Work out the finished part from the listing and answer in its coordinate system (mm). A direction names the side the tool comes from. Give positions to 0.01 mm unless a question says otherwise; leave off trailing zeros. Loops run counter-clockwise (first coordinate to the right, second up) from the corner with the lowest first, then second, coordinate; pieces in that order, holes last. Notation, with made-up numbers: (6, -0.75) -> (60, -0.75) arc R20 cw to (60, 23.25) -> close; hole circle Ø10 at (71.25, -9). An arc over 180 degrees is marked (long way). Answer as CSV lines item,"result". Start each with the question number.
1. Find section D-D, the plane x = 7.5. Give the vertices of the cut face in (y, z).
2. A tool of negligible diameter and unlimited length cuts with its end or side. For faces 5 (the face through (30.758, 2.465, -17.726)), 6 (the face through (2.74, 2.46, 33.43)), 7 (the face through (-27.522, 2.465, -19.077)), 8 (the face through (-30.282, 2.465, 14.296)), 9 (the face through (27.522, 2.465, 19.077)), from which of +Z, -Z, +X, -X, +Y, -Y can it reach the whole face along a straight path? Write none if from no direction.
3. Determine the mould class of faces 1 (the face through (15.59, 2.46, 27.37)), 2 (the face through (27.583, 2.465, -19.088)), 3 (the face through (30.32, 2.46, 14.34)), 4 (the face through (30.282, 2.465, -14.296)) for opening direction Z: +Z half, -Z half, draft (parallel to the pull), parting line (faces both ways), or undercut.
4. Find the intervals of material crossed by line 1 along X through (y, z) = (1.5, 20); line 2 along X through (y, z) = (3.45, -16); line 3 along Z through (x, y) = (-22, 0.25), in increasing order.
5. A flat-ended cylindrical pin translates along its axis: pin 1 Ø1.5 at (y, z) = (2, -2) entering from +X. Find the tip coordinate at first contact, or state that the pin passes through.
6. Find section C-C, the plane z = 4.5. Give the vertices of the cut face in (x, y), and give its area (3 significant figures).
7. Find section B-B, the plane x = 0. Give the vertices of the cut face in (y, z).
8. Find section A-A, the plane y = 3.7. Give the vertices of the cut face in (x, z), and give its area (3 significant figures).
from build123d import *

# Parameters (mm, degrees)
BOSS_EXTRUDE1_DEPTH = 5
SKETCH2_R           = 2.6
CUT_EXTRUDE1_DEPTH  = 5


with BuildPart() as part:
    # Sketch1 → Boss-Extrude1 (new body)
    with BuildSketch(Plane(origin=(0, 0, 0), x_dir=(1, 0, 0), z_dir=(0, 1, 0))):
        with BuildLine():
            Line((2, 35.5), (-2, 35.5))
            Line((-2, 35.5), (-3.5, 31.304951685))
            ThreePointArc((-3.5, 31.304951685), (-15.75, 27.279800219), (-25.360883423, 18.683564756))
            Line((-25.360883423, 18.683564756), (-29.743901834, 19.482050808))
            Line((-29.743901834, 19.482050808), (-31.743901834, 16.017949192))
            Line((-31.743901834, 16.017949192), (-28.860883423, 12.621386929))
            ThreePointArc((-28.860883423, 12.621386929), (-31.5, 0), (-28.860883423, -12.621386929))
            Line((-28.860883423, -12.621386929), (-31.743901834, -16.017949192))
            Line((-31.743901834, -16.017949192), (-29.743901834, -19.482050808))
            Line((-29.743901834, -19.482050808), (-25.360883423, -18.683564756))
            ThreePointArc((-25.360883423, -18.683564756), (-15.75, -27.279800219), (-3.5, -31.304951685))
            Line((-3.5, -31.304951685), (-2, -35.5))
            Line((-2, -35.5), (2, -35.5))
            Line((2, -35.5), (3.5, -31.304951685))
            ThreePointArc((3.5, -31.304951685), (15.75, -27.279800219), (25.360883423, -18.683564756))
            Line((25.360883423, -18.683564756), (29.743901834, -19.482050808))
            Line((29.743901834, -19.482050808), (31.743901834, -16.017949192))
            Line((31.743901834, -16.017949192), (28.860883423, -12.621386929))
            ThreePointArc((28.860883423, -12.621386929), (31.5, 0), (28.860883423, 12.621386929))
            Line((28.860883423, 12.621386929), (31.743901834, 16.017949192))
            Line((31.743901834, 16.017949192), (29.743901834, 19.482050808))
            Line((29.743901834, 19.482050808), (25.360883423, 18.683564756))
            ThreePointArc((25.360883423, 18.683564756), (15.75, 27.279800219), (3.5, 31.304951685))
            Line((3.5, 31.304951685), (2, 35.5))
        make_face()
    extrude(amount=BOSS_EXTRUDE1_DEPTH)

    # Sketch2 → Cut-Extrude1 (cut)
    with BuildSketch(Plane(origin=(0, 5, 0), x_dir=(1, 0, 0), z_dir=(0, 1, 0))):
        with Locations(Location((0, 20, 0), (0, 0, 270))):
            Circle(SKETCH2_R)
        with Locations(Location((0, -20, 0), (0, 0, 90))):
            Circle(SKETCH2_R)
    extrude(amount=-CUT_EXTRUDE1_DEPTH, mode=Mode.SUBTRACT)


solid = part.part
Resolved:
1,outline,"(0, -30.59) -> (5, -30.59) -> (5, 30.59) -> (0, 30.59) -> close"
2,face 5,"-Z, +X, +Y, -Y"
2,face 6,"+Z, +X, +Y, -Y"
2,face 7,"-Z, +Y, -Y"
2,face 8,"-X, +Y, -Y"
2,face 9,"+Z, +Y, -Y"
3,face 1,"+Z half"
3,face 2,"-Z half"
3,face 3,"undercut"
3,face 4,"undercut"
4,line 1,"x = -24.34 to -2.6, 2.6 to 24.34"
4,line 2,"x = -31.73 to 31.73"
4,line 3,"z = -22.54 to 22.54"
5,pin 1,"stops at x = 31.48"
6,outline,"(-31.18, 0) -> (31.18, 0) -> (31.18, 5) -> (-31.18, 5) -> close"
6,area,"312 mm^2"
7,outline,"(0, -35.5) -> (5, -35.5) -> (5, -22.6) -> (0, -22.6) -> close; (0, -17.4) -> (5, -17.4) -> (5, 17.4) -> (0, 17.4) -> close; (0, 22.6) -> (5, 22.6) -> (5, 35.5) -> (0, 35.5) -> close"
8,outline,"(-31.74, -16.02) -> (-29.74, -19.48) -> (-25.36, -18.68) arc R31.5 ccw to (-3.5, -31.3) -> (-2, -35.5) -> (2, -35.5) -> (3.5, -31.3) arc R31.5 ccw to (25.36, -18.68) -> (29.74, -19.48) -> (31.74, -16.02) -> (28.86, -12.62) arc R31.5 ccw to (28.86, 12.62) -> (31.74, 16.02) -> (29.74, 19.48) -> (25.36, 18.68) arc R31.5 ccw to (3.5, 31.3) -> (2, 35.5) -> (-2, 35.5) -> (-3.5, 31.3) arc R31.5 ccw to (-25.36, 18.68) -> (-29.74, 19.48) -> (-31.74, 16.02) -> (-28.86, 12.62) arc R31.5 ccw to (-28.86, -12.62) -> close; hole circle Ø5.2 at (0, -20); hole circle Ø5.2 at (0, 20)"
8,area,"3,210 mm^2"
